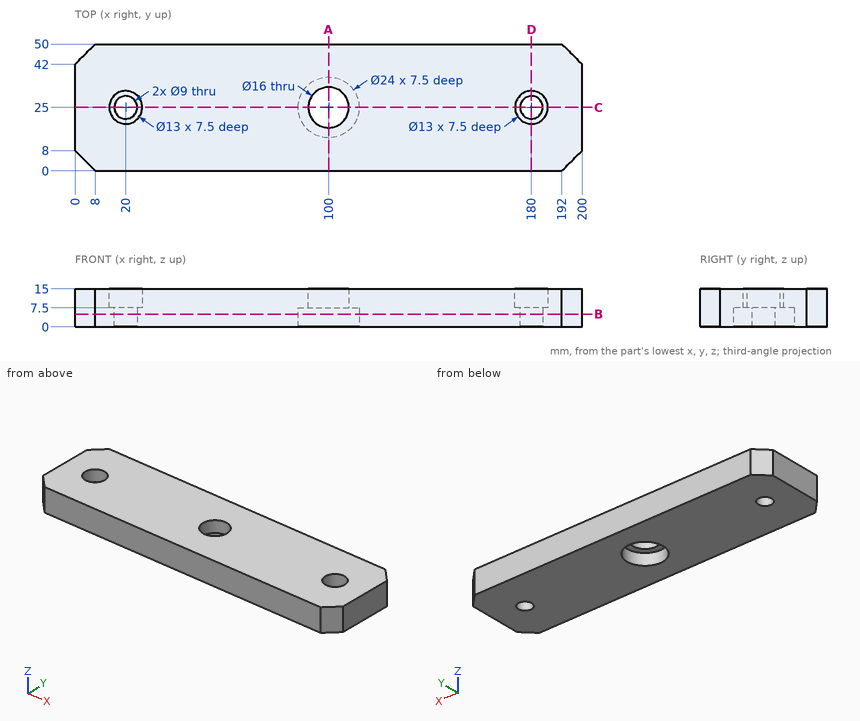
The drawing under review shows one solid part. Ordinate dimensions are in mm from its lowest x, y, z. Give positions to 0.01 mm unless a question says otherwise; leave off trailing zeros. Order: outer loops, then holes, each group sorted by start corner. A loop starts at its lowest first (then second) coordinate and runs counter-clockwise, first axis right, second up. Notation, with made-up numbers: (58.5, 82) -> (111.5, 82) arc R17 ccw to (111.5, 102) -> close; hole circle Ø4 at (88, -33.5). An arc over 180 degrees is marked (long way). Write item = value, one per line. Start each with the question number.
(1) We need section C-C on y = 25. Write out the cut boundary in (x, z).
(2) To check wall thickness, follow line 1 along Y through (x, z) = (20, 12.5); line 2 along Y through (x, z) = (180, 5.5); line 3 along X through (y, z) = (30, 10.5) (3 decimals). State the ranges of each line that lie inside material, in increasing order.
(3) For pin 1 (7 mm diameter, centred on x = 103.5, y = 28, fed in from -Z); pin 2 (11.5 mm diameter, centred on x = 180, y = 25, fed in from -Z); pin 3 (4 mm diameter, centred on x = 17.5, y = 26, fed in from +Z), all flat-tipped, find the tip position at first contact; note any pin that passes through.
(4) We need section B-B on z = 5. Write out the cut boundary in (x, y).
(5) We need section A-A on x = 100. Write out the cut boundary in (y, z).
(6) We need section D-D on x = 180. Write out the cut boundary in (y, z), plus the area to 3 significant figures.
Numbers:
q1.outline = (0, 0) -> (15.5, 0) -> (15.5, 7.5) -> (13.5, 7.5) -> (13.5, 15) -> (0, 15) -> close; (24.5, 0) -> (88, 0) -> (88, 7.5) -> (92, 7.5) -> (92, 15) -> (26.5, 15) -> (26.5, 7.5) -> (24.5, 7.5) -> close; (108, 7.5) -> (112, 7.5) -> (112, 0) -> (175.5, 0) -> (175.5, 7.5) -> (173.5, 7.5) -> (173.5, 15) -> (108, 15) -> close; (184.5, 0) -> (200, 0) -> (200, 15) -> (186.5, 15) -> (186.5, 7.5) -> (184.5, 7.5) -> close
q2.line_1 = 0 to 18.5, 31.5 to 50
q2.line_2 = 0 to 20.5, 29.5 to 50
q2.line_3 = 0 to 15.847, 24.153 to 93.755, 106.245 to 175.847, 184.153 to 200
q3.pin_1 = 7.5
q3.pin_2 = 0
q3.pin_3 = 7.5
q4.outline = (0, 8) -> (8, 0) -> (192, 0) -> (200, 8) -> (200, 42) -> (192, 50) -> (8, 50) -> (0, 42) -> close; hole circle Ø9 at (20, 25); hole circle Ø24 at (100, 25); hole circle Ø9 at (180, 25)
q5.outline = (0, 0) -> (13, 0) -> (13, 7.5) -> (17, 7.5) -> (17, 15) -> (0, 15) -> close; (33, 7.5) -> (37, 7.5) -> (37, 0) -> (50, 0) -> (50, 15) -> (33, 15) -> close
q6.outline = (0, 0) -> (20.5, 0) -> (20.5, 7.5) -> (18.5, 7.5) -> (18.5, 15) -> (0, 15) -> close; (29.5, 0) -> (50, 0) -> (50, 15) -> (31.5, 15) -> (31.5, 7.5) -> (29.5, 7.5) -> close
q6.area = 585 mm^2
